The model under review builds one solid part; all positions refer to its coordinate system, in mm. Face numbers are marked on the shaded views. Round coordinates to 2 decimals unless told otherwise and drop trailing zeros. Write each loop counter-clockwise with the first axis right and the second up, starting at its lowest first coordinate (ties: lowest second). Pieces come first, ordered by that corner, then holes. Notation, with made-up numbers: M 28.25,-25.75 L 43.25,-25.75 A34 ccw 43.25,11.25 Z; hole C 89,86.25 d8. An arc over 180 degrees is marked long. Write item = value, one per line. Start each with the question number.
Item 1: To check wall thickness, follow line 1 along X through (y, z) = (12, -38); line 2 along X through (y, z) = (18, 0); line 3 along X through (y, z) = (19.2, 9.5). State the ranges of each line that lie inside material, in increasing order.
Item 2: Take a section at B-B, the plane y = 6.5. Give the boundary of the cut face in (x, z), plus the area to 3 significant figures.
Item 3: Take a section at C-C, the plane z = -34. Give the boundary of the cut face in (x, y).
Item 4: For pin 1 Ø1.5 at (y, z) = (18, -21.5) entering from -X; pin 2 Ø0.7 at (y, z) = (11.5, -39) entering from +X; pin 3 Ø12 at (y, z) = (7, 0) entering from -X, all flat-tipped, find the tip position at first contact; note any pin that passes through.
Item 5: The part is to be moulded in two halves that separate along X. For the marked faces 1, 2 and 3, say which applies: +X half, -X half, draft (parallel to the pull), parting line (faces both ways), or undercut.
Item 6: Take a section at D-D, the plane z = 9.5. Give the boundary of the cut face in (x, y), plus the area to 3 significant figures.
Item 7: Take a section at A-A, the plane x = 26. Give the boundary of the cut face in (y, z), plus the area to 3 significant figures.
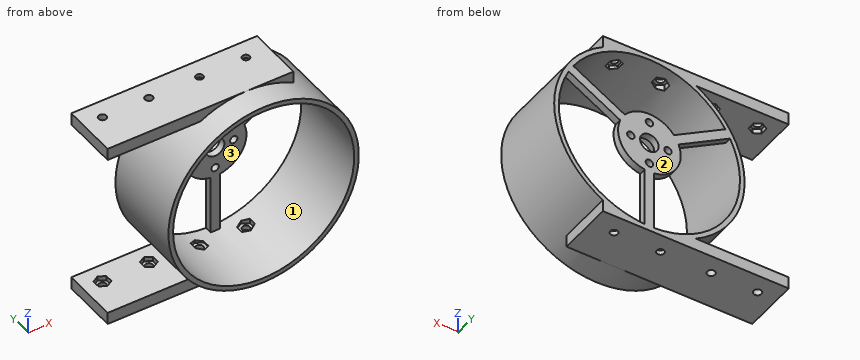
from build123d import *

# Parameters (mm, degrees)
SKETCH_1_R           = 41
SKETCH_1_R_2         = 39
EXTRUDE_1_DEPTH      = 20
EXTRUDE_START        = -14
EXTRUDE_2_DEPTH      = 14
EXTRUDE_START_2      = -3
SKETCH_3_R           = 4
SKETCH_3_R_2         = 1.6
EXTRUDE_3_DEPTH      = 3
CUT_EXTRUDE_3_DEPTH  = 3
EXTRUDE_5_DEPTH      = 10
EXTRUDE_5_DEPTH_BACK = 15
SKETCH_1_2_R         = 41
SKETCH_1_2_R_2       = 39
EXTRUDE_START_3      = 10
EXTRUDE_7_DEPTH      = 10
EXTRUDE_8_DEPTH      = 10
EXTRUDE_8_DEPTH_BACK = 5
CUT_EXTRUDE_4_DEPTH  = 80
EXTRUDE_START_4      = -24
EXTRUDE_10_DEPTH     = 24
EXTRUDE_9_DEPTH      = 10
EXTRUDE_9_DEPTH_BACK = 1.5
CUT_EXTRUDE_6_DEPTH  = 10
SKETCH_16_R          = 1.6
CUT_EXTRUDE_7_DEPTH  = 103
SKETCH_18_R          = 1.6
CUT_EXTRUDE_8_DEPTH  = 10
SKETCH_18_4_R        = 1.6
CUT_EXTRUDE_9_DEPTH  = 10
SKETCH_21_W          = 5.208939664
SKETCH_21_H          = 24
EXTRUDE_11_DEPTH     = 40
SKETCH_22_W          = 5.208939664
SKETCH_22_H          = 24
EXTRUDE_12_DEPTH     = 40
SKETCH_23_R          = 1.7
CUT_EXTRUDE_10_DEPTH = 10
CUT_EXTRUDE_START    = -2
SKETCH_24_R          = 1.7
CUT_EXTRUDE_11_DEPTH = 2


# Read off the part's stored shape, not the designer's step: the extrude step
with BuildPart() as part:
    # 草图1 → 凸台-拉伸1 (new body)
    with BuildSketch(Plane(origin=(0, 0, 0), x_dir=(1, 0, 0), z_dir=(0, 1, 0))):
        with Locations(Location((0, 0, 0), (0, 0, 270))):
            Circle(SKETCH_1_R)
        with Locations(Location((0, 0, 0), (0, 0, 270))):
            Circle(SKETCH_1_R_2, mode=Mode.SUBTRACT)
    extrude(amount=EXTRUDE_1_DEPTH)

    # 草图2 → 凸台-拉伸2 (add)
    with BuildSketch(Plane(origin=(0, 20, 0), x_dir=(1, 0, 0), z_dir=(0, 1, 0)).offset(EXTRUDE_START)):
        with BuildLine():
            Line((-20, -41), (3.5e-08, -41))
            ThreePointArc((3.5e-08, -41), (-10.333598732, -39.676400256), (-20, -35.791060336))
            Line((-20, -35.791060336), (-20, -41))
        make_face()
        with BuildLine():
            Line((3.5e-08, -41), (20, -41))
            Line((20, -41), (20, -35.791060336))
            ThreePointArc((20, -35.791060336), (10.333598766, -39.676400247), (3.5e-08, -41))
        make_face()
    extrude(amount=EXTRUDE_2_DEPTH)

    # 草图3 → 凸台-拉伸3 (add)
    with BuildSketch(Plane(origin=(0, 20, 0), x_dir=(1, 0, 0), z_dir=(0, 1, 0)).offset(EXTRUDE_START_2)):
        with BuildLine():
            Line((-2, 38.948684188), (-2, 13.351029923))
            ThreePointArc((-2, 13.351029923), (-11.691342951, 6.75), (-12.56233108, -4.943464154))
            Line((-12.56233108, -4.943464154), (-34.730549951, -17.742291287))
            ThreePointArc((-34.730549951, -17.742291287), (-33.774990748, -19.5), (-32.730549951, -21.206392902))
            Line((-32.730549951, -21.206392902), (-10.56233108, -8.407565769))
            ThreePointArc((-10.56233108, -8.407565769), (0, -13.5), (10.56233108, -8.407565769))
            Line((10.56233108, -8.407565769), (32.730549951, -21.206392902))
            ThreePointArc((32.730549951, -21.206392902), (33.774990748, -19.5), (34.730549951, -17.742291287))
            Line((34.730549951, -17.742291287), (12.56233108, -4.943464154))
            ThreePointArc((12.56233108, -4.943464154), (11.691342951, 6.75), (2, 13.351029923))
            Line((2, 13.351029923), (2, 38.948684188))
            ThreePointArc((2, 38.948684188), (0, 39), (-2, 38.948684188))
        make_face()
        with Locations(Location((0, 0, 0), (0, 0, 270))):
            Circle(SKETCH_3_R, mode=Mode.SUBTRACT)
        with Locations(Location((-8, 0, 0), (0, 0, 270))):
            Circle(SKETCH_3_R_2, mode=Mode.SUBTRACT)
        with Locations(Location((8, 0, 0), (0, 0, 270))):
            Circle(SKETCH_3_R_2, mode=Mode.SUBTRACT)
    extrude(amount=EXTRUDE_3_DEPTH)

    # 草图7 → 切除-拉伸3 (cut)
    with BuildSketch(Plane.XZ.offset(-6)):
        with BuildLine():
            Line((0, 41), (-20, 41))
            Line((-20, 41), (-20, 35.791060336))
            ThreePointArc((-20, 35.791060336), (-10.333598749, 39.676400251), (0, 41))
        make_face()
        with BuildLine():
            Line((20, 41), (0, 41))
            ThreePointArc((0, 41), (10.333598749, 39.676400251), (20, 35.791060336))
            Line((20, 35.791060336), (20, 41))
        make_face()
    extrude(amount=-CUT_EXTRUDE_3_DEPTH, mode=Mode.SUBTRACT)

    # 草图1<2> → 凸台-拉伸5 (add, two sides: drawn at the far end of the back side and taken through both)
    with BuildSketch(Plane(origin=(0, 0, 0), x_dir=(1, 0, 0), z_dir=(0, 1, 0)).offset(-EXTRUDE_5_DEPTH_BACK)):
        with Locations(Location((0, 0, 0), (0, 0, 270))):
            Circle(SKETCH_1_2_R)
        with Locations(Location((0, 0, 0), (0, 0, 92.939534486))):
            Circle(SKETCH_1_2_R_2, mode=Mode.SUBTRACT)
    extrude(amount=EXTRUDE_5_DEPTH + EXTRUDE_5_DEPTH_BACK)

    # 草图7<4> → 凸台-拉伸7 (add)
    with BuildSketch(Plane.XZ.offset(-6).offset(EXTRUDE_START_3)):
        with BuildLine():
            Line((0, 41), (-20, 41))
            Line((-20, 41), (-20, 35.791060336))
            ThreePointArc((-20, 35.791060336), (-10.333598749, 39.676400251), (0, 41))
        make_face()
        with BuildLine():
            Line((20, 41), (0, 41))
            ThreePointArc((0, 41), (10.333598749, 39.676400251), (20, 35.791060336))
            Line((20, 35.791060336), (20, 41))
        make_face()
    extrude(amount=-EXTRUDE_7_DEPTH)

    # 草图7<5> → 凸台-拉伸8 (add, two sides: drawn at the far end of the back side and taken through both)
    with BuildSketch(Plane.XZ.offset(-6).offset(-EXTRUDE_8_DEPTH_BACK)):
        with BuildLine():
            Line((0, 41), (-20, 41))
            Line((-20, 41), (-20, 35.791060336))
            ThreePointArc((-20, 35.791060336), (-10.333598749, 39.676400251), (0, 41))
        make_face()
        with BuildLine():
            Line((20, 41), (0, 41))
            ThreePointArc((0, 41), (10.333598749, 39.676400251), (20, 35.791060336))
            Line((20, 35.791060336), (20, 41))
        make_face()
    extrude(amount=EXTRUDE_8_DEPTH + EXTRUDE_8_DEPTH_BACK)

    # 草图4 → 切除-拉伸4 (cut)
    with BuildSketch(Plane.XY.offset(41)):
        Polygon((-10, 8.766838493), (-7.2, 10.383419246), (-7.2, 13.616580754), (-10, 15.233161507), (-12.8, 13.616580754), (-12.8, 10.383419246), align=None)
        Polygon((12.8, 10.383419246), (10, 8.766838493), (7.2, 10.383419246), (7.2, 13.616580754), (10, 15.233161507), (12.8, 13.616580754), align=None)
    extrude(amount=-CUT_EXTRUDE_4_DEPTH, mode=Mode.SUBTRACT)

    # 凸台-拉伸10 outline → 凸台-拉伸10 (add)
    with BuildSketch(Plane(origin=(0, 20, 0), x_dir=(1, 0, 0), z_dir=(0, 1, 0)).offset(EXTRUDE_START_4)):
        with BuildLine():
            Line((20, 35.791060336), (20, 41))
            Line((20, 41), (8e-08, 41))
            ThreePointArc((8e-08, 41), (6.403124277, 40.496913456), (12.649110641, 39))
            ThreePointArc((12.649110641, 39), (12.72457916, 38.975442079), (12.8, 38.950738119))
            ThreePointArc((12.8, 38.950738119), (16.475918515, 37.543895763), (20, 35.791060336))
        make_face()
        with BuildLine():
            ThreePointArc((-12.649110641, 39), (-6.403124198, 40.496913469), (8e-08, 41))
            Line((8e-08, 41), (-20, 41))
            Line((-20, 41), (-20, 35.791060336))
            ThreePointArc((-20, 35.791060336), (-16.475918515, 37.543895763), (-12.8, 38.950738119))
            ThreePointArc((-12.8, 38.950738119), (-12.72457916, 38.975442079), (-12.649110641, 39))
        make_face()
    extrude(amount=EXTRUDE_10_DEPTH)

    # 草图4<3> → 凸台-拉伸9 (add, two sides: drawn at the far end of the back side and taken through both)
    with BuildSketch(Plane.XY.offset(41).offset(-EXTRUDE_9_DEPTH_BACK)):
        Polygon((-10, 8.766838493), (-7.2, 10.383419246), (-7.2, 13.616580754), (-10, 15.233161507), (-12.8, 13.616580754), (-12.8, 10.383419246), align=None)
        Polygon((12.8, 10.383419246), (10, 8.766838493), (7.2, 10.383419246), (7.2, 13.616580754), (10, 15.233161507), (12.8, 13.616580754), align=None)
    extrude(amount=EXTRUDE_9_DEPTH + EXTRUDE_9_DEPTH_BACK)

    # 草图13 → 切除-拉伸6 (cut)
    with BuildSketch(Plane.XY.offset(51)):
        Polygon((10, 15.233161507), (7.2, 13.616580754), (7.2, 10.383419246), (10, 8.766838493), (12.8, 10.383419246), (12.8, 13.616580754), align=None)
        Polygon((-10, 15.233161507), (-12.8, 13.616580754), (-12.8, 10.383419246), (-10, 8.766838493), (-7.2, 10.383419246), (-7.2, 13.616580754), align=None)
    extrude(amount=-CUT_EXTRUDE_6_DEPTH, mode=Mode.SUBTRACT)

    # 草图16 → 切除-拉伸7 (cut)
    with BuildSketch(Plane.XY.offset(41)):
        with Locations((-10, 12)):
            Circle(SKETCH_16_R)
        with Locations((10, 12)):
            Circle(SKETCH_16_R)
    extrude(amount=-CUT_EXTRUDE_7_DEPTH, mode=Mode.SUBTRACT)

    # 草图18 → 切除-拉伸8 (cut)
    with BuildSketch(Plane(origin=(0, 20, 0), x_dir=(1, 0, 0), z_dir=(0, 1, 0))):
        with Locations(Location((0, 9.5, 0), (0, 0, 270))):
            Circle(SKETCH_18_R)
    extrude(amount=-CUT_EXTRUDE_8_DEPTH, mode=Mode.SUBTRACT)

    # 草图18<4> → 切除-拉伸9 (cut)
    with BuildSketch(Plane(origin=(0, 20, 0), x_dir=(1, 0, 0), z_dir=(0, 1, 0))):
        with Locations(Location((0, 9.5, 0), (0, 0, 270))):
            Circle(SKETCH_18_4_R)
        with Locations(Location((0, -9.5, 0), (0, 0, 270))):
            Circle(SKETCH_18_4_R)
    extrude(amount=-CUT_EXTRUDE_9_DEPTH, mode=Mode.SUBTRACT)

    # 草图21 → 凸台-拉伸11 (add)
    with BuildSketch(Plane.ZY.offset(20)):
        with Locations((38.395530168, 8)):
            Rectangle(SKETCH_21_W, SKETCH_21_H)
    extrude(amount=EXTRUDE_11_DEPTH)

    # 草图22 → 凸台-拉伸12 (add)
    with BuildSketch(Plane.ZY.offset(20)):
        with Locations((-38.395530168, 8)):
            Rectangle(SKETCH_22_W, SKETCH_22_H)
    extrude(amount=EXTRUDE_12_DEPTH)

    # 草图23 → 切除-拉伸10 (cut)
    with BuildSketch(Plane.XY.offset(41)):
        with Locations((-51.796444508, 12)):
            Circle(SKETCH_23_R)
        with Locations((-31.796444508, 12)):
            Circle(SKETCH_23_R)
    cut_extrude_10 = extrude(amount=-CUT_EXTRUDE_10_DEPTH, mode=Mode.SUBTRACT)

    # 草图24 → 切除-拉伸11 (cut)
    # profile 1 of 2: a face of its own
    with BuildSketch(Plane(origin=(0, 0, 35.791060336), x_dir=(-1, 0, 0), z_dir=(0, 0, -1)).offset(CUT_EXTRUDE_START)):
        Polygon((28.996444508, 10.340970788), (31.833205951, 8.745614264), (34.633205951, 10.404643475), (34.596444508, 13.659029212), (31.759683065, 15.254385736), (28.959683065, 13.595356525), align=None)
        with Locations(Location((31.796444508, 12, 0), (0, 0, 180))):
            Circle(SKETCH_24_R, mode=Mode.SUBTRACT)
    # profile 2 of 2: a face of its own
    with BuildSketch(Plane(origin=(0, 0, 35.791060336), x_dir=(-1, 0, 0), z_dir=(0, 0, -1)).offset(CUT_EXTRUDE_START)):
        Polygon((51.759683065, 8.745614264), (54.596444508, 10.340970788), (54.633205951, 13.595356525), (51.833205951, 15.254385736), (48.996444508, 13.659029212), (48.959683065, 10.404643475), align=None)
        with Locations(Location((51.796444508, 12, 0), (0, 0, 180))):
            Circle(SKETCH_24_R, mode=Mode.SUBTRACT)
    cut_extrude_11 = extrude(amount=CUT_EXTRUDE_11_DEPTH, mode=Mode.SUBTRACT)

    # 镜向1: 切除-拉伸11 across plane
    add(cut_extrude_11.mirror(Plane(origin=(0, 0, 0), x_dir=(1, 0, 0), z_dir=(0, 0, -1))), mode=Mode.SUBTRACT)

    # 镜向2: 切除-拉伸10 across plane
    add(cut_extrude_10.mirror(Plane(origin=(0, 0, 0), x_dir=(1, 0, 0), z_dir=(0, 0, -1))), mode=Mode.SUBTRACT)


solid = part.part
Response values:
q1.line_1 = -60 to -53.5, -50.1 to -33.5, -30.1 to -12.8, 12.8 to 20
q1.line_2 = -41 to -39, -13.5 to -9.6, -6.4 to -4, 4 to 6.4, 9.6 to 13.5, 39 to 41
q1.line_3 = -39.88 to -37.83, -20.45 to -12.45, -9.59 to -1.6, 1.6 to 9.59, 12.45 to 20.45, 37.83 to 39.88
q2.outline = M -60,-41 L 20,-41 L 20,-35.79 A41 ccw 20,35.79 L 20,41 L -60,41 L -60,35.79 L -20,35.79 A41 ccw -20,-35.79 L -60,-35.79 Z; hole C 0,0 d78
q2.area = 1,050 mm2
q3.outline = M -22.91,-15 L -19.1,-15 L -19.1,20 L -22.91,20 Z; M -2,17 L 2,17 L 2,20 L -2,20 Z; M 19.1,-15 L 22.91,-15 L 22.91,20 L 19.1,20 Z
q4.pin_1 = -35.36
q4.pin_2 = 20
q4.pin_3 = -41
q5.face_1 = undercut
q5.face_2 = draft
q5.face_3 = undercut
q6.outline = M -39.88,-15 L -37.83,-15 L -37.83,20 L -39.88,20 Z; M -20.45,17 L -12.45,17 L -12.45,20 L -20.45,20 Z; M -9.59,17 L -1.6,17 L -1.6,20 L -9.59,20 Z; M 1.6,17 L 9.59,17 L 9.59,20 L 1.6,20 Z; M 12.45,17 L 20.45,17 L 20.45,20 L 12.45,20 Z; M 37.83,-15 L 39.88,-15 L 39.88,20 L 37.83,20 Z
q6.area = 240 mm2
q7.outline = M -15,-31.7 L 20,-31.7 L 20,-29.07 L -15,-29.07 Z; M -15,29.07 L 20,29.07 L 20,31.7 L -15,31.7 Z; M 17,12.7 L 20,12.7 L 20,17.32 L 17,17.32 Z
q7.area = 198 mm2
